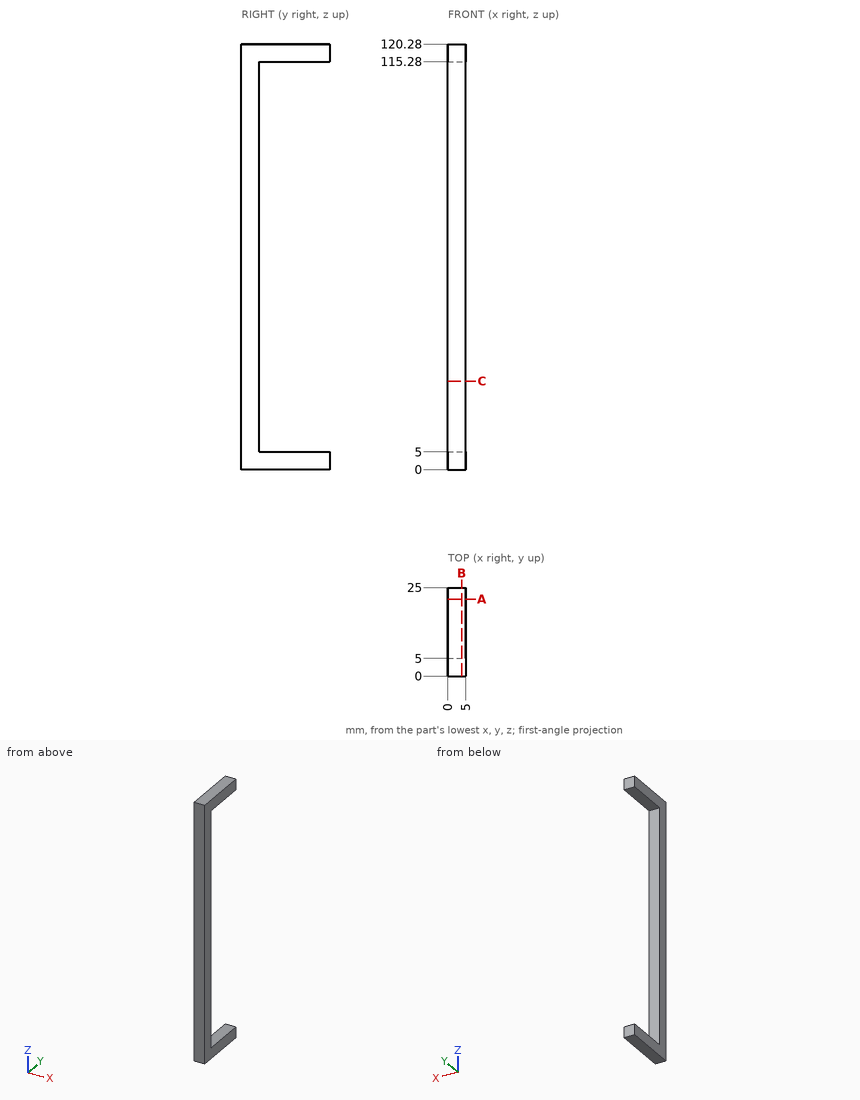
Print and shaded views of the part. All mm, measured from the part's lowest x, y and z. Round coordinates to 2 decimals unless told otherwise and drop trailing zeros. Order: outer loops, then holes, each group sorted by start corner. A loop starts at its lowest first (then second) coordinate and runs counter-clockwise, first axis right, second up.
Q1. Slice it at C-C (z = 25). Write the cut outline in (x, y), and give its area (3 significant figures).
Q2. Drop flat-ended pins along their axis: pin 1 (1 mm diameter, centred on x = 2, z = 65.5, fed in from +Y); pin 2 (3 mm diameter, centred on y = 7.5, z = 91.5, fed in from +X). Give the stop position or say it passes through.
Q3. Slice it at B-B (x = 3.85). Write the cut outline in (y, z).
Q4. Wall check: L1, parallel to Z at x = 2.6, y = 5.25; L2, parallel to Y at x = 2.5, z = 21.5. Give the ranges that are in metal, low to high.
Q5. Slice it at A-A (y = 21.75). Write the cut outline in (x, z), and give its area (3 significant figures).
Results below:
1. outline: (0, 0) - (5, 0) - (5, 5) - (0, 5) - close
1. area: 25.0 mm2
2. pin 1: stops at y = 5
2. pin 2: passes through
3. outline: (0, 0) - (25, 0) - (25, 5) - (5, 5) - (5, 115.28) - (25, 115.28) - (25, 120.28) - (0, 120.28) - close
4. L1: z = 0 to 5, 115.28 to 120.28
4. L2: y = 0 to 5
5. outline: (0, 0) - (5, 0) - (5, 5) - (0, 5) - close; (0, 115.28) - (5, 115.28) - (5, 120.28) - (0, 120.28) - close
5. area: 50.0 mm2
